Autodesk Inventor part; units mm, degrees
ref_plane "YZ Plane" through (0, 0, 0) normal (1, 0, 0) x (0, 1, 0)
ref_plane "XZ Plane" through (0, 0, 0) normal (0, 1, 0) x (-1, 0, 0)
ref_plane "XY Plane" through (0, 0, 0) normal (0, 0, 1) x (1, 0, 0)
sketch "Sketch1" plane through (0, 0, 0) normal (0, 0, 1) x (1, 0, 0)
  arc A0 (6.0987, 0.8622) -> (22, 22) centre (0, 22) ccw
  line L0 (22, 22) -> (22, 37)
  arc A1 (22, 37) -> (13, 54.7482) centre (0, 37) ccw
  line L1 (13, 54.7482) -> (13, 66.7482)
  line L2 (22.5, 90) -> (22.5, 66.7482)
  line L3 (22.5, 90) -> (37.5, 90)
  line L4 (13, 66.7482) -> (22.5, 66.7482)
  line L5 (2.6116, 0) -> (27.6759, 0)
  line L6 (32.3216, 3.1515) -> (37.1457, 15.2755)
  arc A2 (37.1457, 15.2755) -> (37.5, 17.1241) centre (32.5, 17.1241) ccw
  arc A3 (27.6759, 0) -> (32.3216, 3.1515) centre (27.6759, 5) ccw
  line L7 (37.5, 53.562) -> (30, 53.562)
  line L8 (30, 53.562) -> (30, 48.362)
  line L9 (30, 48.362) -> (37.5, 48.362)
  line L10 (37.5, 43.362) -> (30, 43.362)
  line L11 (30, 43.362) -> (30, 38.162)
  line L12 (30, 38.162) -> (37.5, 38.162)
  line L13 (37.5, 90) -> (37.5, 53.562)
  line L14 (37.5, 48.362) -> (37.5, 43.362)
  line L15 (37.5, 38.162) -> (37.5, 17.1241)
  line L16 (6.0987, 0.8622) -> (2.6116, 0)
  point P0 (0, 0)
  dimension "d0" = 22
  dimension "d1" = 90
  dimension "d2" = 0
  dimension "d3" = 15
  dimension "d4" = 0
  dimension "d5" = 13
  dimension "d6" = 22
  dimension "d7" = 12
  dimension "d8" = 22.5
  dimension "d10" = 90
  dimension "d11" = 37
  dimension "d12" = 5
  dimension "d13" = 12.1241
  dimension "d14" = 5.2
  dimension "d15" = 5.2
  dimension "d16" = 5
sketch "Sketch2" plane through (0, 0, 0) normal (0, 0, 1) x (1, 0, 0)
  point P0 (0, 0)
extrude "Extrusion1" add sketch "Sketch1" along normal blind 5
sketch "Sketch3" plane through (0, 0, 5) normal (0, 0, 1) x (1, 0, 0)
  line L0 (22.5, 90) -> (22.5, 66.7482)
  line L1 (37.5, 90) -> (22.5, 90)
  point P0 (0, 0)
  point P1 (30, 86.5)
  point P2 (30, 68.5)
  dimension "d20" = 18
  dimension "d21" = 7.5
  dimension "d22" = 7.5
  dimension "d23" = 3.5
hole "Hole1" at (30, 86.5, 5) at (30, 68.5, 5) direction (0, 0, -1) diameter 3.4 end through all
sketch "Sketch4" plane through (22.5, 66.7482, 0) normal (-1, 0, 0) x (0, 0, 1)
  line L0 (-7.9102, 0) -> (13.3435, 0)
  line L1 (13.3435, 0) -> (13.3435, 24.2425)
  line L2 (13.3435, 24.2425) -> (-7.9102, 24.2425)
  line L3 (-7.9102, 24.2425) -> (-7.9102, 0)
  line L4 (0, 0) -> (5, 0)
  point P0 (0, -66.7482)
  dimension "d31" = 0
extrude "Extrusion2" cut sketch "Sketch4" against normal blind 15
sketch "Sketch5" plane through (13, 54.7482, 0) normal (-1, 0, 0) x (0, 0, 1)
  line L0 (-8.9151, 14.3214) -> (15.4889, 14.3214)
  line L1 (15.4889, 14.3214) -> (15.4889, 5)
  line L2 (15.4889, 5) -> (-8.9151, 5)
  line L3 (-8.9151, 5) -> (-8.9151, 14.3214)
  line L4 (0, 12) -> (5, 12)
  point P0 (0, -54.7482)
  dimension "d34" = 7
extrude "Extrusion3" cut sketch "Sketch5" against normal blind 40
properties part number "Finger"
Verification items for the finished model (mm, model axes). A direction names the side the tool comes from. Coordinates: 2 decimals unless noted, no trailing zeros. Order: outer loops, then holes, each group sorted by start corner. A loop starts at its lowest first (then second) coordinate and runs counter-clockwise, first axis right, second up.
1. Sectioned sample at B-B, the plane z = 2.1. Record the cut outline in (x, y).
Results found:
outline: (2.61, 0) - (27.68, 0) arc R5 ccw to (32.32, 3.15) - (37.15, 15.28) arc R5 ccw to (37.5, 17.12) - (37.5, 38.16) - (30, 38.16) - (30, 43.36) - (37.5, 43.36) - (37.5, 48.36) - (30, 48.36) - (30, 53.56) - (37.5, 53.56) - (37.5, 59.75) - (13, 59.75) - (13, 54.75) arc R22 cw to (22, 37) - (22, 22) arc R22 cw to (6.1, 0.86) - close
2. Scan lines: line 1 (Y direction, x = 32, z = 0.85); line 2 (Y direction, x = 17, z = 1.1); line 3 (Y direction, x = 17.5, z = 0.7). Record each from-to range of solid material in increasing order.
Results found:
line 1: y = 2.49 to 38.16, 43.36 to 48.36, 53.56 to 59.75
line 2: y = 0 to 8.04, 50.96 to 59.75
line 3: y = 0 to 8.67, 50.33 to 59.75
3. Release check for a two-part mould opening along Y. For faces 1 (the face through (34, 43.362, 2)), 2 (the face through (37.413, 16.196, 2.465)), 3 (the face through (13, 57, 2)) record: +Y half, -Y half, draft (parallel to the pull), parting line (faces both ways), or undercut.
Results found:
face 1: undercut
face 2: -Y half
face 3: draft
4. Set-up check for faces 4 (the face through (19.556, 47.079, 2.465)), 5 (the face through (28, 30, 0)), 6 (the face through (34, 53.562, 2)): record each of +Z, -Z, +X, -X, +Y, -Y from which the full face is reachable in a straight line by a thin tool's end or side.
Results found:
face 4: +Z, -Z, -X
face 5: -Z, +X, -X, +Y, -Y
face 6: +Z, -Z, +X
5. Sectioned sample at C-C, the plane y = 29.5. Record the cut outline in (x, z), and give its area (3 significant figures).
Results found:
outline: (22, 0) - (37.5, 0) - (37.5, 5) - (22, 5) - close
area: 77.5 mm2
6. Go/stop test with flat-tipped pins: pin 1 Ø1.5 at (y, z) = (39.5, 1.5) entering from +X; pin 2 Ø6 at (x, y) = (14, 52) entering from -Z; pin 3 Ø2 at (x, z) = (6, 2.5) entering from +Y; pin 4 Ø2.5 at (y, z) = (57.5, 3.5) entering from -X. Record where each tip stops, or that it passes through.
Results found:
pin 1: stops at x = 30
pin 2: stops at z = 0
pin 3: stops at y = 1.14
pin 4: stops at x = 13
7. Sectioned sample at D-D, the plane x = 14. Record the cut outline in (y, z), and give its area (3 significant figures).
Results found:
outline: (0, 0) - (5.03, 0) - (5.03, 5) - (0, 5) - close; (53.97, 0) - (59.75, 0) - (59.75, 5) - (53.97, 5) - close
area: 54.0 mm2
8. Sectioned sample at A-A, the plane x = 19.5. Record the cut outline in (y, z).
Results found:
outline: (0, 0) - (11.81, 0) - (11.81, 5) - (0, 5) - close; (47.19, 0) - (59.75, 0) - (59.75, 5) - (47.19, 5) - close
